Part model, mm, in its own coordinate system. Round coordinates to 2 decimals unless told otherwise and drop trailing zeros. Loops run counter-clockwise (first coordinate to the right, second up) from the corner with the lowest first, then second, coordinate; pieces in that order, holes last.
(1) Cut at A-A on y = 0. List the corners of the cut face in (x, z).
(2) Flat gauge pins, fed straight in: pin 1 (23.5 mm diameter, centred on x = -17.5, y = -37.5, fed in from -Z); pin 2 (0.5 mm diameter, centred on x = 8, z = 0.5, fed in from +Y); pin 3 (0.8 mm diameter, centred on x = 14.5, z = 0.5, fed in from -Y); pin 4 (1 mm diameter, centred on x = 9, z = 0, fed in from +Y). Where does each tip first touch, or does it go through?
(3) Cut at B-B on z = 1.3. List the corners of the cut face in (x, y).
(4) Cut at C-C on y = 59.5. List the corners of the cut face in (x, z), then the cut area to 3 significant figures.
(5) Probe probe 1 along Y at (x, z) = (0, 1.65); probe 2 along Y at (x, z) = (-17, 1.8); probe 3 along X at (y, z) = (32, 1.45). List the from-to ranges inside material, lowest first.
from build123d import *

# Parameters (mm, degrees)
SKETCH1_R           = 70
SKETCH1_R_2         = 36
BOSS_EXTRUDE1_DEPTH = 2
CUT_EXTRUDE1_DEPTH  = 1
CIRPATTERN1_COUNT   = 18


with BuildPart() as part:
    # Sketch1 → Boss-Extrude1 (new body)
    with BuildSketch(Plane.XY):
        Circle(SKETCH1_R)
        Circle(SKETCH1_R_2, mode=Mode.SUBTRACT)
    extrude(amount=BOSS_EXTRUDE1_DEPTH)

    # Sketch2 → Cut-Extrude1 (cut)
    with BuildSketch(Plane.XY):
        with BuildLine():
            Line((-41, 40.5), (3, 40.5))
            ThreePointArc((3, 40.5), (3.5, 40), (3, 39.5))
            Line((3, 39.5), (-41, 39.5))
            ThreePointArc((-41, 39.5), (-41.5, 40), (-41, 40.5))
        make_face()
    cut_extrude1 = extrude(amount=CUT_EXTRUDE1_DEPTH, mode=Mode.SUBTRACT)

    # CirPattern1: Cut-Extrude1 ×18 about axis
    cirpattern1_axis = Axis((0, 0, 0), (0, 0, 1))
    for i in range(1, CIRPATTERN1_COUNT):
        add(cut_extrude1.rotate(cirpattern1_axis, i * 360 / CIRPATTERN1_COUNT), mode=Mode.SUBTRACT)


solid = part.part
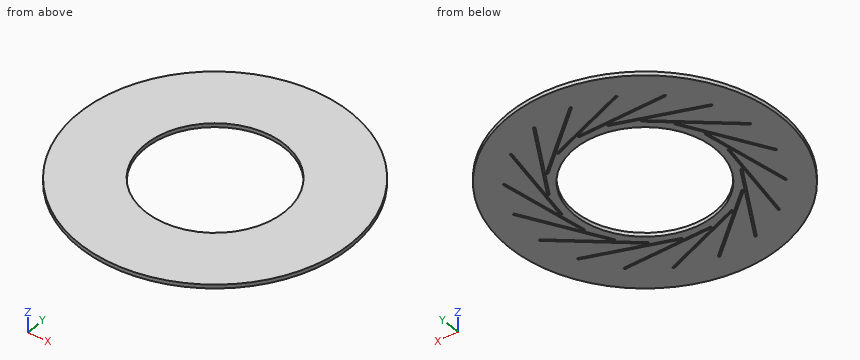
Final values:
1. outline: (-70, 0) - (-46.77, 0) - (-46.77, 1) - (-45.61, 1) - (-45.61, 0) - (-41.12, 0) - (-41.12, 1) - (-40.11, 1) - (-40.11, 0) - (-36, 0) - (-36, 2) - (-70, 2) - close; (36, 0) - (40.11, 0) - (40.11, 1) - (41.12, 1) - (41.12, 0) - (45.61, 0) - (45.61, 1) - (46.77, 1) - (46.77, 0) - (70, 0) - (70, 2) - (36, 2) - close
2. pin 1: stops at z = 0
2. pin 2: stops at y = 69.57
2. pin 3: stops at y = -68.57
2. pin 4: stops at y = 69.48
3. outline: circle Ø140 at (0, 0); hole circle Ø72 at (0, 0)
4. outline: (-36.87, 0) - (36.87, 0) - (36.87, 2) - (-36.87, 2) - close
4. area: 147 mm2
5. probe 1: y = -70 to -36, 36 to 70
5. probe 2: y = -67.9 to -31.73, 31.73 to 67.9
5. probe 3: x = -62.26 to -16.49, 16.49 to 62.26
